from build123d import *

# Parameters (mm, degrees)
CYLINDER980_R     = 1
CYLINDER980_DEPTH = 20
CYLINDER977_R     = 1
CYLINDER977_DEPTH = 20
CYLINDER976_R     = 1
CYLINDER976_DEPTH = 20
CYLINDER979_R     = 1
CYLINDER979_DEPTH = 20
TUBE092_R         = 9
TUBE092_R_2       = 2.8
TUBE092_DEPTH     = 10


with BuildPart() as obj1:
    # Cylinder980 → Cylinder980 (new body)
    with BuildSketch(Plane(origin=(4.5, -4.5, -88), x_dir=(0, 1, 0), z_dir=(0, 0, 1))):
        Circle(CYLINDER980_R)
    extrude(amount=CYLINDER980_DEPTH)


with BuildPart() as obj2:
    # Cylinder977 → Cylinder977 (new body)
    with BuildSketch(Plane(origin=(4.5, 4.5, -88), x_dir=(-1, 0, 0), z_dir=(0, 0, 1))):
        Circle(CYLINDER977_R)
    extrude(amount=CYLINDER977_DEPTH)


with BuildPart() as obj3:
    # Cylinder976 → Cylinder976 (new body)
    with BuildSketch(Plane(origin=(-4.5, 4.5, -88), x_dir=(0, -1, 0), z_dir=(0, 0, 1))):
        Circle(CYLINDER976_R)
    extrude(amount=CYLINDER976_DEPTH)


with BuildPart() as compound809:
    # Cylinder979 → Cylinder979 (new body)
    with BuildSketch(Plane(origin=(-4.5, -4.5, -88), x_dir=(1, 0, 0), z_dir=(0, 0, 1))):
        Circle(CYLINDER979_R)
    extrude(amount=CYLINDER979_DEPTH)

    # Compound809: union obj1, obj2, obj3
    add(obj1.part)
    add(obj2.part)
    add(obj3.part)


with BuildPart() as compound809_1:
    # Compound809 placement: moved
    add(compound809.part.moved(Location((0, 0, 91))))


with BuildPart() as cut413:
    # Tube092 → Tube092 (new body)
    with BuildSketch(Plane.XY.offset(19)):
        Circle(TUBE092_R)
        Circle(TUBE092_R_2, mode=Mode.SUBTRACT)
    extrude(amount=TUBE092_DEPTH)

    # Cut413: cut Compound809
    add(compound809_1.part, mode=Mode.SUBTRACT)


solid = cut413.part
Work out the finished part from the listing and answer in its coordinate system (mm). A direction names the side the tool comes from. Round coordinates to 2 decimals unless told otherwise and drop trailing zeros. Write each loop counter-clockwise with the first axis right and the second up, starting at its lowest first coordinate (ties: lowest second). Pieces come first, ordered by that corner, then holes. Notation, with made-up numbers: (71.25, -21.75) -> (78.25, -21.75) arc R4 ccw to (78.25, -15.75) -> close; hole circle Ø6 at (-3.5, 3.25). An arc over 180 degrees is marked (long way). Write each question's results on one line, items separated by ' | '.
Item 1: A cutting plane is placed at B-B, the plane z = 20.5. Determine the outline of the cut face in (x, y).
Result set:
outline: circle Ø18 at (0, 0); hole circle Ø2 at (-4.5, -4.5); hole circle Ø2 at (-4.5, 4.5); hole circle Ø5.6 at (0, 0); hole circle Ø2 at (4.5, -4.5); hole circle Ø2 at (4.5, 4.5)
Item 2: A cutting plane is placed at D-D, the plane y = 4.75. Determine the outline of the cut face in (x, z).
Result set:
outline: (-7.64, 19) -> (-5.47, 19) -> (-5.47, 23) -> (-3.53, 23) -> (-3.53, 19) -> (3.53, 19) -> (3.53, 23) -> (5.47, 23) -> (5.47, 19) -> (7.64, 19) -> (7.64, 29) -> (-7.64, 29) -> close
Item 3: Flat-ended cylindrical pins translate along their axes: P1, Ø1.8, axis at x = 4.5, y = -4.5, coming from the -Z side; P2, Ø1, axis at x = 4, z = 21, coming from the +Y side; P3, Ø4, axis at y = -0.5, z = 24.5, coming from the -X side; P4, Ø2, axis at x = -5.5, z = 24, coming from the -Y side. Find the tip coordinate at first contact, or state that the pin passes through.
Result set:
P1: z = 23 | P2: y = 8.29 | P3: x = -9 | P4: y = -7.79
Item 4: The mould has two halves that part along Y. Classify faces 1 (the face through (4, -5, 23)), 2 (the face through (-1.172, 8.923, 23.93)), 3 (the face through (-2.8, 0.1, 23.9)), 4 (the face through (-2.1, 2.1, 19)): +Y half, -Y half, draft (parallel to the pull), parting line (faces both ways), or undercut.
Result set:
face 1: undercut | face 2: parting line | face 3: undercut | face 4: draft
Item 5: A cutting plane is placed at A-A, the plane x = 0. Determine the outline of the cut face in (y, z), plus the area to 3 significant figures.
Result set:
outline: (-9, 19) -> (-2.8, 19) -> (-2.8, 29) -> (-9, 29) -> close; (2.8, 19) -> (9, 19) -> (9, 29) -> (2.8, 29) -> close | area: 124 mm^2
Item 6: Which of the six approach directions +Z, -Z, +X, -X, +Y, -Y give full straight-line access (tool end or side, diameter ignored) to faces 5 (the face through (-3.51, 4.63, 20.97)), 6 (the face through (-2.1, 2.1, 29))?
Result set:
face 5: -Z | face 6: +Z, +X, -X, +Y, -Y
Item 7: Find the intervals of material crossed by line 1 along X through (y, z) = (-4.5, 21); line 2 along Y through (x, z) = (3.75, 22), in increasing order. Write a range as [from, to].
Result set:
line 1: [-7.79, -5.5], [-3.5, 3.5], [5.5, 7.79] | line 2: [-8.18, -5.16], [-3.84, 3.84], [5.16, 8.18]
